from build123d import *

# Parameters (mm, degrees)
GUIDE_BUSH_BARREL_SKETCH_R      = 6
GUIDE_BUSH_BARREL_DEPTH         = 10
GUIDE_BUSH_FLANGE_SKETCH_R      = 7
GUIDE_BUSH_FLANGE_DEPTH         = 1.05
DIRECTIONAL_RUNNING_SLOT_DEPTH  = 11.25
ANTIROTATION_GUIDE_KEY_SKETCH_W = 1.3
ANTIROTATION_GUIDE_KEY_SKETCH_H = 1.2
ANTIROTATION_GUIDE_KEY_DEPTH    = 8
MOVE2_ANGLE                     = 120


with BuildPart() as part:
    # Guide bush barrel sketch → Guide bush barrel (new body)
    with BuildSketch(Plane(origin=(0, -105.98, 0), x_dir=(1, 0, 0), z_dir=(0, 1, 0))):
        with Locations(Location((-20.291651246, 0, 0), (0, 0, 270))):
            Circle(GUIDE_BUSH_BARREL_SKETCH_R)
    extrude(amount=GUIDE_BUSH_BARREL_DEPTH)

    # Guide bush flange sketch → Guide bush flange (add)
    with BuildSketch(Plane(origin=(0, -95.98, 0), x_dir=(1, 0, 0), z_dir=(0, 1, 0))):
        with Locations(Location((-20.291651246, 0, 0), (0, 0, 270))):
            Circle(GUIDE_BUSH_FLANGE_SKETCH_R)
    extrude(amount=GUIDE_BUSH_FLANGE_DEPTH)

    # Directional running slot sketch → Directional running slot (cut)
    with BuildSketch(Plane(origin=(0, -106.08, 0), x_dir=(1, 0, 0), z_dir=(0, 1, 0))):
        with BuildLine():
            Line((-23.086458867, -4.240748797), (-22.566843625, -4.540748797))
            ThreePointArc((-22.566843625, -4.540748797), (-15.641094828, -2.685), (-17.496843625, 4.240748797))
            Line((-17.496843625, 4.240748797), (-18.016458867, 4.540748797))
            ThreePointArc((-18.016458867, 4.540748797), (-24.942207664, 2.685), (-23.086458867, -4.240748797))
        make_face()
    extrude(amount=DIRECTIONAL_RUNNING_SLOT_DEPTH, mode=Mode.SUBTRACT)

    # Antirotation guide key sketch → Antirotation guide key (add)
    with BuildSketch(Plane(origin=(0, -105, 0), x_dir=(1, 0, 0), z_dir=(0, 1, 0))):
        with Locations((-13.841651246, 0)):
            Rectangle(ANTIROTATION_GUIDE_KEY_SKETCH_W, ANTIROTATION_GUIDE_KEY_SKETCH_H)
    extrude(amount=ANTIROTATION_GUIDE_KEY_DEPTH)


with BuildPart() as part_1:
    # Move1: moved
    add(part.part.moved(Location((56.291651246, 0, 0))))


with BuildPart() as part_2:
    # Move2: moved
    add(part_1.part.rotate(Axis((0, 0, 0), (0, -1, 0)), MOVE2_ANGLE))


with BuildPart() as part_3:
    # Move3: moved
    add(part_2.part.moved(Location((-56.291651246, 0, 0))))


with BuildPart() as body_2:
    # Mirror1: mirrored copy
    add(part_3.part.mirror(Plane(origin=(0, 0, 0), x_dir=(0, 0, 1), z_dir=(0, -1, 0))))


solid = body_2.part
Input: part model. Units: mm. Frame: model coordinates. A direction names the side the tool comes from. Round coordinates to 2 decimals unless told otherwise and drop trailing zeros. Order: outer loops, then holes, each group sorted by start corner. A loop starts at its lowest first (then second) coordinate and runs counter-clockwise, first axis right, second up. Notation, with made-up numbers: (-24.75, -34) - (16.25, -34) arc R25 cw to (16.25, -2) - close; hole circle Ø3 at (-39.75, 34). An arc over 180 degrees is marked (long way). Answer as a JSON object with one key per item and string values. Group by question number.
(1) Reachability of faces 4 (the face through (-77.036, 101.056, 37.13)), 5 (the face through (-78, 105, 37)), 6 (the face through (-79, 100.53, 33.76)), 7 (the face through (-78.075, 101.056, 36.53)), 8 (the face through (-78, 97, 37)) from +Z, -Z, +X, -X, +Y, -Y: full face, straight path, thin tool, end or side. Return the list, or none.
(2) Cut plane B-B (x = -76). Return loops of the section in (y, z).
(3) Pin query (flat end, axial travel): P1, Ø2, axis at x = -73, z = 36, coming from the +Y side; P2, Ø5, axis at x = -72, y = 100, coming from the +Z side; P3, Ø6, axis at y = 100.5, z = 34, coming from the +X side; P4, Ø1, axis at x = -72, y = 97.5, coming from the -Z side. Return the tip coordinate at first contact, or that it passes through.
(4) Cut plane C-C (z = 29). Return loops of the section in (x, y).
(5) Material intervals for probe 1 along X at (y, z) = (104.5, 31.25); probe 2 along Y at (x, z) = (-69.75, 36.25); probe 3 along Z at (x, y) = (-78, 105.25), sorted ascending. Write a range as from..to.
(6) Cut plane D-D (x = -78). Return loops of the section in (y, z).
(7) Draft query along Z for faces 1 (the face through (-69.586, 100.532, 28.589)), 2 (the face through (-76, 94.93, 26)), 3 (the face through (-77.85, 101.06, 37.32)). Return one class per face: released by +Z, released by -Z, zero draft, split by the parting line, or undercut.
Here are the results:
{
 "1": {"face 4": "+Z, +Y", "face 5": "+Z, -X, +Y", "face 6": "+Y, -Y", "face 7": "-X, +Y", "face 8": "+Z, -X"},
 "2": {"outline": "(94.93, 24.39) - (95.98, 24.39) - (95.98, 25.43) - (105.98, 25.43) - (105.98, 26.35) - (94.93, 26.35) - close; (94.93, 36.19) - (105.98, 36.19) - (105.98, 36.93) - (95.98, 36.93) - (95.98, 37.97) - (94.93, 37.97) - close"},
 "3": {"P1": "stops at y = 105.98", "P2": "stops at z = 37.18", "P3": "stops at x = -68.29", "P4": "stops at z = 25.45"},
 "4": {"outline": "(-80.94, 94.93) - (-79.06, 94.93) - (-79.06, 105.98) - (-79.88, 105.98) - (-79.88, 95.98) - (-80.94, 95.98) - close; (-69.38, 94.93) - (-67.64, 94.93) - (-67.64, 95.98) - (-68.7, 95.98) - (-68.7, 105.98) - (-69.38, 105.98) - close"},
 "5": {"probe 1": "x = -80.29..-79.62, -68.97..-68.29", "probe 2": "y = 94.93..95.98", "probe 3": "z = 26.46..27.61, 35.04..35.89"},
 "6": {"outline": "(94.93, 25.24) - (95.98, 25.24) - (95.98, 26.46) - (105.98, 26.46) - (105.98, 27.61) - (94.93, 27.61) - close; (94.93, 35.04) - (105.98, 35.04) - (105.98, 35.89) - (95.98, 35.89) - (95.98, 37.11) - (94.93, 37.11) - close; (97, 36.4) - (105, 36.4) - (105, 37.23) - (97, 37.23) - close"},
 "7": {"face 1": "undercut", "face 2": "zero draft", "face 3": "released by +Z"}
}
